```python
from build123d import *

# Parameters (mm, degrees)
SKETCH1_W           = 24
SKETCH1_H           = 48
BOSS_EXTRUDE1_DEPTH = 8
FILLET2_R           = 4
SKETCH2_R           = 2.5
CUT_EXTRUDE1_DEPTH  = 8
FILLET3_R           = 1


with BuildPart() as part:
    # Sketch1 → Boss-Extrude1 (new body)
    with BuildSketch(Plane(origin=(0, 0, 0), x_dir=(1, 0, 0), z_dir=(0, 1, 0))):
        Rectangle(SKETCH1_W, SKETCH1_H)
    extrude(amount=BOSS_EXTRUDE1_DEPTH)

    # Fillet2
    fillet2_edges = [part.edges().sort_by_distance(p)[0] for p in [
        (-12, 4, 24),
        (-12, 4, -24),
        (12, 4, -24),
        (12, 4, 24),
    ]]
    fillet(fillet2_edges, radius=FILLET2_R)

    # Sketch2 → Cut-Extrude1 (cut)
    with BuildSketch(Plane(origin=(0, 8, 0), x_dir=(1, 0, 0), z_dir=(0, 1, 0))):
        with Locations(Location((8, -12, 0), (0, 0, 270))):
            Circle(SKETCH2_R)
        with Locations(Location((-8, -12, 0), (0, 0, 270))):
            Circle(SKETCH2_R)
    extrude(amount=-CUT_EXTRUDE1_DEPTH, mode=Mode.SUBTRACT)

    # Fillet3
    fillet3_edges = [part.edges().sort_by_distance(p)[0] for p in [
        (0, 0, 24),
        (0, 8, 24),
        (-12, 0, 0),
        (0, 0, -24),
        (12, 0, 0),
        (10.828427125, 0, -22.828427125),
        (10.828427125, 0, 22.828427125),
        (-10.828427125, 0, -22.828427125),
        (-10.828427125, 0, 22.828427125),
        (-12, 8, 0),
        (12, 8, 0),
        (0, 8, -24),
        (10.828427125, 8, -22.828427125),
        (10.828427125, 8, 22.828427125),
        (-10.828427125, 8, -22.828427125),
        (-10.828427125, 8, 22.828427125),
    ]]
    fillet(fillet3_edges, radius=FILLET3_R)


solid = part.part
```
For this review, take the finished solid that the model builds, in its own axes (mm). Give positions to 0.01 mm unless a question says otherwise; leave off trailing zeros. Order: outer loops, then holes, each group sorted by start corner. A loop starts at its lowest first (then second) coordinate and runs counter-clockwise, first axis right, second up.
1) Take a section at C-C (x = 7.5). Give the boundary of the cut face in (y, z).
2) The part is to be moulded in two halves that separate along Z. For faces 1 (the face through (-10.859, 4.042, 22.797)), 2 (the face through (-9.5, 4.1, 10)), 3 (the face through (11.699, 0.285, -0.28)), 4 (the face through (5.56, 4.06, 11.46)), say which applies: released by +Z, released by -Z, zero draft, split by the parting line, or undercut.
3) Wall thickness on line 1 (X direction, y = 4.5, z = 12); line 2 (Z direction, x = -10, y = 5.5); line 3 (Z direction, x = 5.75, y = 1): over which ranges is each line inside the solid? List them lowest first.
4) Insertion check: pin 1 (5 mm diameter, centred on x = -8, z = 13, fed in from -Y). The pin has a flat end and moves straight along its axis. Give the tip position at first contact, or say it passes through.
5) Take a section at B-B (y = 6.25). Give the boundary of the cut face in (x, z), then the cut area to 3 significant figures.
6) Take a section at A-A (z = 12). Give the boundary of the cut face in (x, y), then the cut area to 3 significant figures.
Derived:
1. outline: (0, -23) arc R1 ccw to (1, -24) - (7, -24) arc R1 ccw to (8, -23) - (8, 9.55) - (0, 9.55) - close; (0, 14.45) - (8, 14.45) - (8, 23) arc R1 ccw to (7, 24) - (1, 24) arc R1 ccw to (0, 23) - close
2. face 1: released by +Z
2. face 2: undercut
2. face 3: zero draft
2. face 4: undercut
3. line 1: x = -12 to -10.5, -5.5 to 5.5, 10.5 to 12
3. line 2: z = -23.46 to 10.5, 13.5 to 23.46
3. line 3: z = -24 to 10.91, 13.09 to 24
4. pin 1: stops at y = 0
5. outline: (-12, -20) arc R4 ccw to (-8, -24) - (8, -24) arc R4 ccw to (12, -20) - (12, 20) arc R4 ccw to (8, 24) - (-8, 24) arc R4 ccw to (-12, 20) - close; hole circle Ø5 at (-8, 12); hole circle Ø5 at (8, 12)
5. area: 1,100 mm2
6. outline: (-12, 1) arc R1 ccw to (-11, 0) - (-10.5, 0) - (-10.5, 8) - (-11, 8) arc R1 ccw to (-12, 7) - close; (-5.5, 0) - (5.5, 0) - (5.5, 8) - (-5.5, 8) - close; (10.5, 0) - (11, 0) arc R1 ccw to (12, 1) - (12, 7) arc R1 ccw to (11, 8) - (10.5, 8) - close
6. area: 111 mm2
